Here's the drawing with two shaded views (mm, measured from the low corner). I have some questions. A direction names the side the tool comes from. Coordinates: 2 decimals unless noted, no trailing zeros. Loops run counter-clockwise (first coordinate to the right, second up) from the corner with the lowest first, then second, coordinate; pieces in that order, holes last. Notation, with made-up numbers: M 70,-13 L 78,-13 A18 ccw 78,21 Z; hole C 13.25,37 d8. An arc over 180 degrees is marked long. Use one line per item in the form item = value. Start each with the question number.
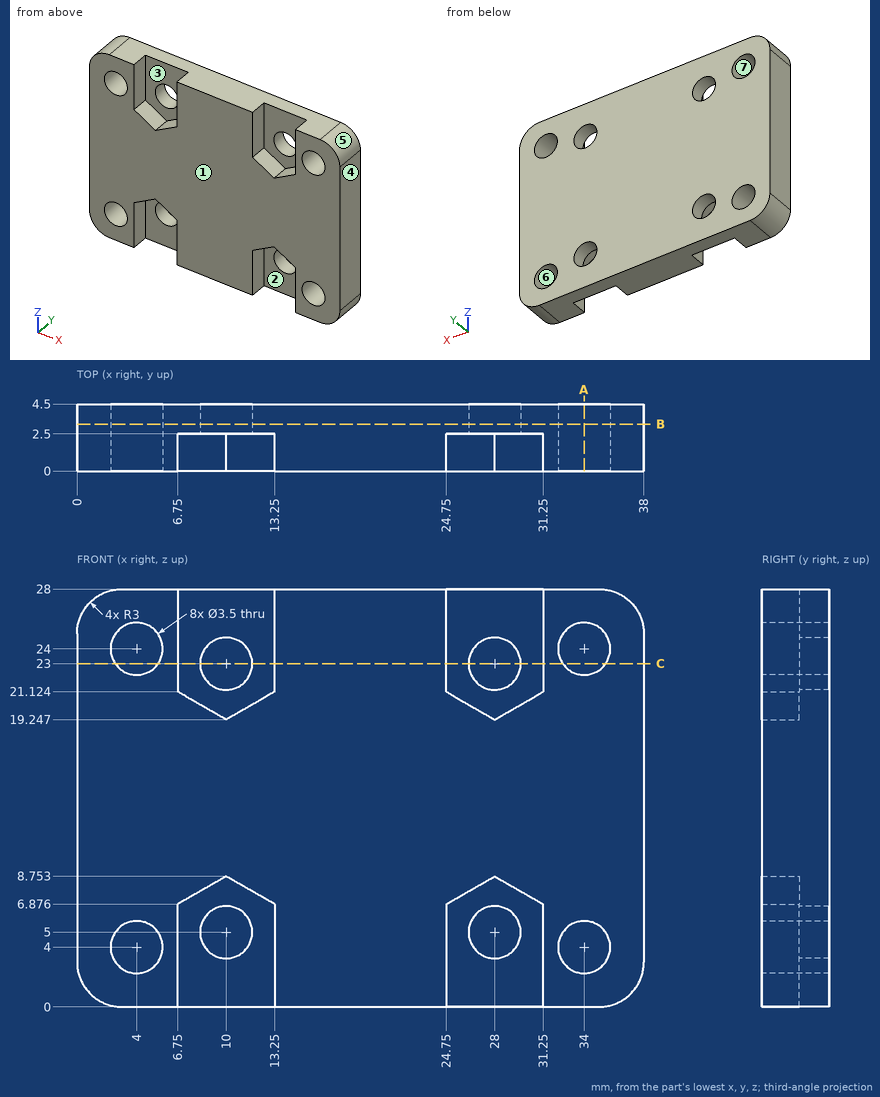
Item 1: I want a section at A-A (x = 34). Write out the boundary of the cut face in (y, z).
Item 2: Thinking about a two-plate mould opening in Z: for the marked faces 4, 5, 6 and 7, which applies, pulls with the +Z half, pulls with the -Z half, needs draft (parallel to the pull), parting line crosses it, or undercut?
Item 3: I want a section at B-B (y = 3.15). Count the separate pieces of the cut face and the enclosed holes in it, plus the area to 3 significant figures.
Item 4: For the marked faces 1, 2 and 3, which set-ups out of +Z, -Z, +X, -X, +Y, -Y let a thin tool reach every point of the face, with its end or its side?
Item 5: Please list where these lines run through material, in increasing order: line 1 along Z through (x, y) = (34, 2.55); line 2 along Z through (x, y) = (28, 3.6); line 3 along X through (y, z) = (1.5, 4).
Item 6: I'm going to push flat-ended pins straight in: P1, Ø4, axis at x = 10, z = 5, coming from the -Y side; P2, Ø3, axis at x = 34, z = 4, coming from the -Y side; P3, Ø0.8, axis at y = 0.5, z = 2, coming from the -X side. Where does each tip first touch, or does it pass through?
Item 7: I want a section at C-C (z = 23). Write out the boundary of the cut face in (x, y).
Worked answers:
q1.outline = M 0,0 L 4.5,0 L 4.5,2.25 L 0,2.25 Z; M 0,5.75 L 4.5,5.75 L 4.5,22.25 L 0,22.25 Z; M 0,25.75 L 4.5,25.75 L 4.5,28 L 0,28 Z
q2.face_4 = needs draft
q2.face_5 = pulls with the +Z half
q2.face_6 = undercut
q2.face_7 = undercut
q3.separate_pieces = 1
q3.enclosed_holes = 8
q3.area = 979 mm²
q4.face_1 = +Z, -Z, +X, -X, -Y
q4.face_2 = -Z, -Y
q4.face_3 = +Z, -Y
q5.line_1 = 0 to 2.25, 5.75 to 22.25, 25.75 to 28
q5.line_2 = 0 to 3.25, 6.75 to 21.25, 24.75 to 28
q5.line_3 = 0 to 2.25, 5.75 to 6.75, 13.25 to 24.75, 31.25 to 32.25, 35.75 to 38
q6.P1 = 2.5
q6.P2 = through
q6.P3 = 0.06
q7.outline = M 0,0 L 2.56,0 L 2.56,4.5 L 0,4.5 Z; M 5.44,0 L 6.75,0 L 6.75,2.5 L 8.25,2.5 L 8.25,4.5 L 5.44,4.5 Z; M 11.75,2.5 L 13.25,2.5 L 13.25,0 L 24.75,0 L 24.75,2.5 L 26.25,2.5 L 26.25,4.5 L 11.75,4.5 Z; M 29.75,2.5 L 31.25,2.5 L 31.25,0 L 32.56,0 L 32.56,4.5 L 29.75,4.5 Z; M 35.44,0 L 38,0 L 38,4.5 L 35.44,4.5 Z
